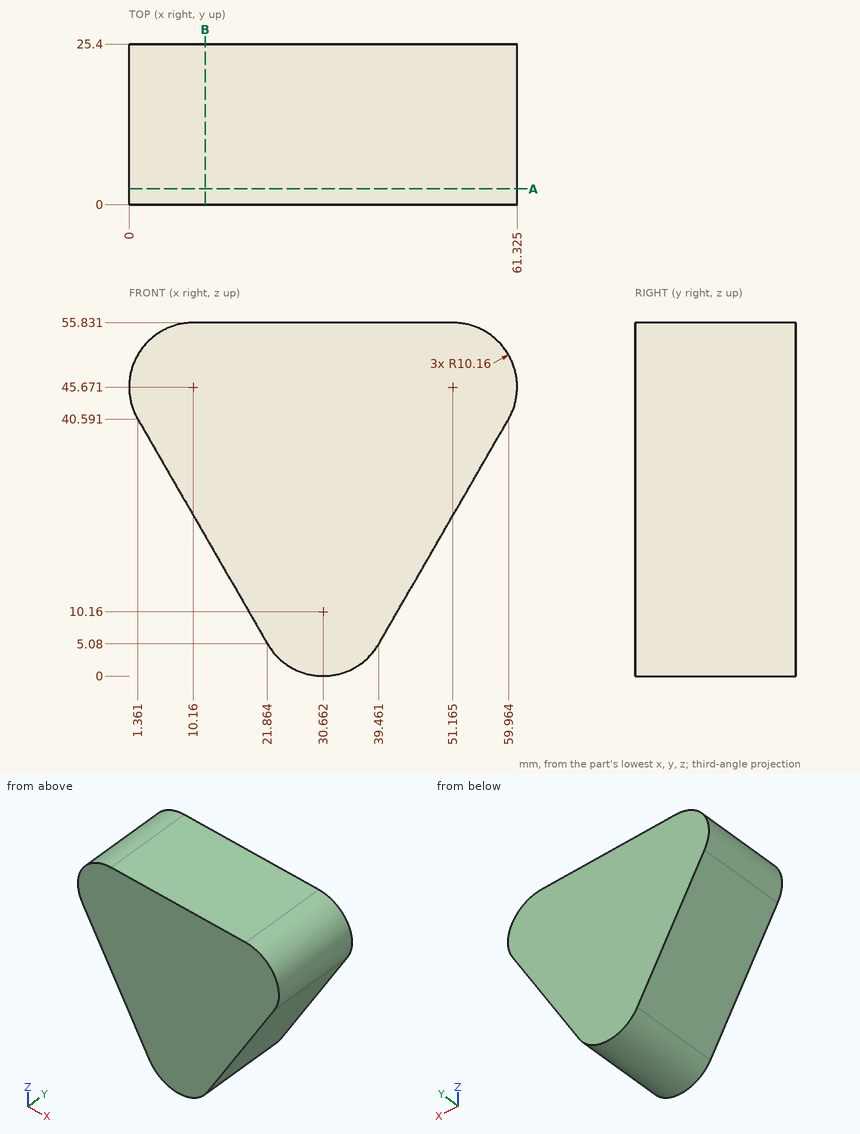
The figure shows three views and two pictorial views of one solid part (mm, origin at its lowest corner). Answer the questions. Give positions to 0.01 mm unless a question says otherwise; leave off trailing zeros. Loops run counter-clockwise (first coordinate to the right, second up) from the corner with the lowest first, then second, coordinate; pieces in that order, holes last. Notation, with made-up numbers: (46, -27) -> (73, -27) arc R22 cw to (73, 12) -> close; hole circle Ø2 at (-26.75, 81). An arc over 180 degrees is marked (long way). Use CSV: the item, a comma, the result in double quotes.
1. Flat-ended cylindrical pins translate along their axes: pin 1 Ø8 at (y, z) = (18, 19) entering from -X; pin 2 Ø5 at (x, y) = (43, 22.5) entering from -Z; pin 3 Ø6 at (y, z) = (15, 9) entering from +X. Find the tip coordinate at first contact, or state that the pin passes through.
Found:
pin 1,"x = 11.52"
pin 2,"z = 6.88"
pin 3,"x = 43.46"
2. The part is cut by section A-A (y = 2.5). Write down the section's boundary in (x, z) (1 decimal), then the cut area to 3 significant figures.
Found:
outline,"(1.4, 40.6) -> (21.9, 5.1) arc R10.2 ccw to (39.5, 5.1) -> (60, 40.6) arc R10.2 ccw to (51.2, 55.8) -> (10.2, 55.8) arc R10.2 ccw to start"
area,"2,300 mm^2"
3. Straight lines are drawn through the part: line 1 (Z direction, x = 25, y = 2.25) (1 decimal); line 2 (Z direction, x = 57, y = 4.5) (1 decimal); line 3 (X direction, y = 10.75, z = 25). For each, find the intervals that lie inside material, in ascending order.
Found:
line 1,"1.7 to 55.8"
line 2,"35.5 to 54"
line 3,"10.36 to 50.96"
4. The part is cut by section B-B (x = 12). Write down the section's boundary in (y, z) (1 decimal), then the cut area to 3 significant figures.
Found:
outline,"(0, 22.2) -> (25.4, 22.2) -> (25.4, 55.8) -> (0, 55.8) -> close"
area,"855 mm^2"
